Build history of the part. All positions in model axes, mm. A direction names the side the tool comes from. Give positions to 0.01 mm unless a question says otherwise; leave off trailing zeros. Loops run counter-clockwise (first coordinate to the right, second up) from the corner with the lowest first, then second, coordinate; pieces in that order, holes last. Notation, with made-up numbers: (88, 60.5) - (131, 60.5) arc R13 ccw to (131, 64.5) - close; hole circle Ø10 at (60.5, 3). An arc over 180 degrees is marked (long way). Return JSON: item names as keys, results as strings. Group by question number.
1) Slice it at B-B (z = 45.5). List the corners of the cut face in (x, y).
2) Drill centre lines: probe 1 along Y at (x, z) = (0, 79); probe 2 along Y at (x, z) = (-1.75, 9); probe 3 along X at (y, z) = (1.5, 63.5). Where is each one in solid material? Low to high. Write a range as from..to.
3) Drop flat-ended pins along their axis: pin 1 (1.8 mm diameter, centred on x = -1, z = 77.5, fed in from +Y); pin 2 (2 mm diameter, centred on y = 0.5, z = 69, fed in from +X); pin 3 (2 mm diameter, centred on y = -1.5, z = 70, fed in from +X). Give the stop position or say it passes through.
4) 3-axis set-ups, long thin cutter, end or side, ignore diameter. For faces 1 (the face through (0, 0, 87)), 2 (the face through (0, 1.75, 79)): which of +Z, -Z, +X, -X, +Y, -Y reach the whole face in a straight line?
5) Slice it at A-A (x = 0). List the corners of the cut face in (y, z).
```python
from build123d import *

# Parameters (mm, degrees)
SKETCH1_R           = 2.5
BOSS_EXTRUDE1_DEPTH = 87
SKETCH2_W           = 5
SKETCH2_H           = 0.75
CUT_EXTRUDE1_DEPTH  = 16
CHAMFER1_SIZE       = 0.5
CHAMFER2_SIZE       = 0.866025404
CHAMFER2_SIZE_2     = 0.5


with BuildPart() as part:
    # Sketch1 → Boss-Extrude1 (new body)
    with BuildSketch(Plane.XY):
        Circle(SKETCH1_R)
    extrude(amount=BOSS_EXTRUDE1_DEPTH)

    # Sketch2 → Cut-Extrude1 (cut)
    with BuildSketch(Plane.XY.offset(87)):
        with Locations((0, 2.125)):
            Rectangle(SKETCH2_W, SKETCH2_H)
    extrude(amount=-CUT_EXTRUDE1_DEPTH, mode=Mode.SUBTRACT)

    # Chamfer1
    chamfer1_edges = [part.edges().sort_by_distance(p)[0] for p in [
        (-2.5, 0, 0),
        (-0.945147404, -2.314453798, 87),
    ]]
    chamfer(chamfer1_edges, length=CHAMFER1_SIZE)

    # Chamfer2
    # the kernel refuses this chamfer: 0.866025404, 0.5 mm, written as the material it adds along each edge
    with BuildSketch(Plane(origin=(4.025839092, 1.75, 71), x_dir=(0, 0.999813220622208, -0.01932676561269574), z_dir=(-1, 0, 0))) as chamfer2_piece_1_section:
        Polygon((CHAMFER2_SIZE * 0.999813220373, -CHAMFER2_SIZE * 0.0193267656079), (-CHAMFER2_SIZE_2 * 0.0193267656127, -CHAMFER2_SIZE_2 * 0.999813220622), (0, 0), align=None)
    chamfer2_piece_1 = extrude(amount=8.051678185, mode=Mode.PRIVATE)
    chamfer2_piece_1 = chamfer2_piece_1 & Plane(origin=(0, 0, 71.180869941), x_dir=(1, 0, 0), z_dir=(0, 0, -1)) * Cylinder(2.5, 20, mode=Mode.PRIVATE)
    add(chamfer2_piece_1)


solid = part.part
```
Results:
{
 "1": {"outline": "circle Ø5 at (0, 0)"},
 "2": {"probe 1": "-2.5..1.75", "probe 2": "-1.79..1.79", "probe 3": "-2..2"},
 "3": {"pin 1": "y = 1.75", "pin 2": "x = 2.5", "pin 3": "x = 2.45"},
 "4": {"face 1": "+Z, +X, -X, +Y, -Y", "face 2": "+Z, +X, -X, +Y"},
 "5": {"outline": "(-2.5, 0.5) - (-2, 0) - (2, 0) - (2.5, 0.5) - (2.5, 71.07) - (1.75, 71.5) - (1.75, 87) - (-2, 87) - (-2.5, 86.5) - close"}
}
